Input: part model. Units: mm. Frame: model coordinates. A direction names the side the tool comes from. Coordinates: 2 decimals unless noted, no trailing zeros. Order: outer loops, then holes, each group sorted by start corner. A loop starts at its lowest first (then second) coordinate and runs counter-clockwise, first axis right, second up. Notation, with made-up numbers: (81.25, -18.5) -> (109.25, -18.5) arc R35 cw to (109.25, 14.5) -> close; hole circle Ø3 at (87, 37.5). An arc over 180 degrees is marked (long way). One line per question, with ' | ' between items.
```python
from build123d import *

# Parameters (mm, degrees)
BOSS_EXTRUDE1_DEPTH = 0.5
CIRPATTERN10_COUNT  = 3
SKETCH4_W           = 0.1
SKETCH4_H           = 2


with BuildPart() as part:
    # Sketch1 → Revolve1 (revolve)
    with BuildSketch(Plane.XY):
        with BuildLine():
            Line((0, 0), (0, 388))
            add(Edge.make_bspline(
                [(0, 388), (12, 353.463683825), (12, 313.539168354), (12, 274.912097708), (12, 274)],
                knots=[0, 0, 0, 0, 0.976387086, 1, 1, 1, 1], degree=3))
            Line((12, 274), (12, 0))
            Line((12, 0), (0, 0))
        make_face()
    revolve(axis=Axis((0, 0, 0), (0, 1, 0)))

    # Sketch2 → Boss-Extrude1 (add, symmetric)
    with BuildSketch(Plane.XY):
        Polygon((-12, 0), (-52, -40), (-52, -10), (-12, 55), (-9, 55), (-9, 0), align=None)
    boss_extrude1 = extrude(amount=BOSS_EXTRUDE1_DEPTH, both=True)

    # CirPattern10: Boss-Extrude1 ×3 about axis
    cirpattern10_axis = Axis((0, 0, 0), (0, 1, 0))
    for i in range(1, CIRPATTERN10_COUNT):
        add(boss_extrude1.rotate(cirpattern10_axis, i * 360 / CIRPATTERN10_COUNT))

    # Sketch4 → Cut-Revolve1 (revolve, cut)
    with BuildSketch(Plane.XY):
        with Locations((11.95, 71)):
            Rectangle(SKETCH4_W, SKETCH4_H)
        with Locations((11.95, 248)):
            Rectangle(SKETCH4_W, SKETCH4_H)
    revolve(axis=Axis((0, 0, 0), (0, -1, 0)), mode=Mode.SUBTRACT)


solid = part.part
```
1. Ray query, line 1 (X direction, y = 18, z = -2); line 2 (Z direction, x = -1.5, y = 267.5); line 3 (X direction, y = -6.5, z = 32). Return the intervals inside material, ascending. Write a range as [from, to].
Recorded:
line 1: x = [-11.83, 11.83] | line 2: z = [-11.91, 11.91] | line 3: x = [17.9, 19.05]
2. Access query for faces 1 (the face through (15.854, -19.72, -27.474)), 2 (the face through (-32, 8, -0.5)), 3 (the face through (-32, 8, 0.5)), 4 (the face through (16.29, 8.165, 27.216)). Directions: +Z, -Z, +X, -X, +Y, -Y. A direction counts if a zero-diameter tool reaches every point of the face in a straight line with its end or side. Return the directions, or none.
Recorded:
face 1: -X, -Y | face 2: -Z, -X, +Y, -Y | face 3: +Z, -X, +Y, -Y | face 4: +X, +Y, -Y
3. Cut plane A-A, the plane z = 23. Return loops of the section in (x, y), and give its area (3 significant figures).
Recorded:
outline: (12.7, -14.27) -> (13.86, -14.85) -> (13.86, 30.87) -> (12.7, 31.81) -> close | area: 53.0 mm^2
4. Pin query (flat end, axial travel): pin 1 Ø19 at (x, z) = (-3.5, -2) entering from -Y; pin 2 Ø7 at (x, z) = (-5, -5.5) entering from -Y; pin 3 Ø6 at (x, y) = (-11.5, 168) entering from +Z. Return the tip coordinate at first contact, or that it passes through.
Recorded:
pin 1: stops at y = -0.88 | pin 2: stops at y = 0 | pin 3: stops at z = 8.47
5. Cut plane B-B, the plane y = 158.5. Return loops of the section in (x, z), and give its area (3 significant figures).
Recorded:
outline: circle Ø24 at (0, 0) | area: 452 mm^2
6. Cut plane C-C, the plane x = -35. Return loops of the section in (y, z) (3 decimals), and give its area (3 significant figures).
Recorded:
outline: (-23, -0.5) -> (17.625, -0.5) -> (17.625, 0.5) -> (-23, 0.5) -> close | area: 40.6 mm^2
